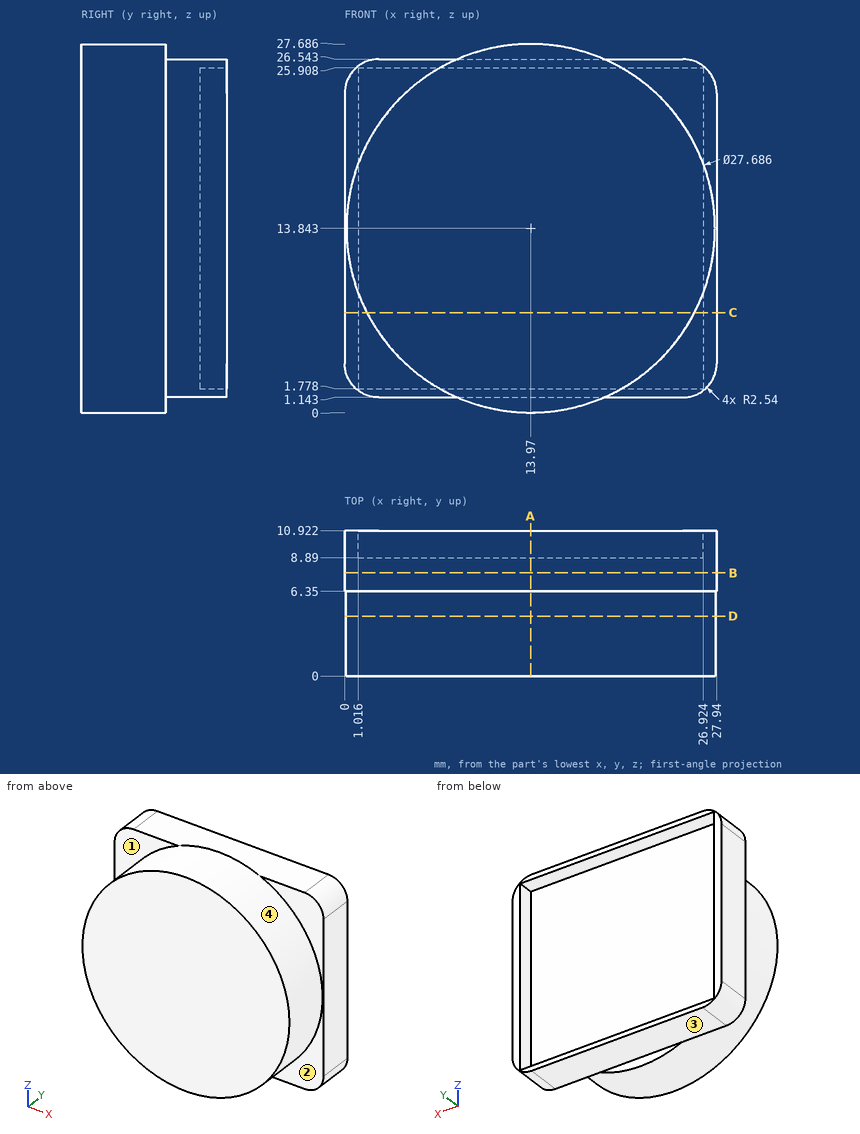
For this review, use the dimensioned drawing (mm, ordinates from the lowest corner) and the shaded views. A direction names the side the tool comes from. Round coordinates to 2 decimals unless told otherwise and drop trailing zeros. Order: outer loops, then holes, each group sorted by start corner. A loop starts at its lowest first (then second) coordinate and runs counter-clockwise, first axis right, second up. Notation, with made-up numbers: M 86.25,-29 L 101.25,-29 A22 cw 101.25,-21 Z; hole C 77,26 d11. An arc over 180 degrees is marked long. Write each question's results on one line, items separated by ' | '. Start each with the question number.
1. Add section B-B (y = 7.75). State the section outline as (x, z) points.
2. To check wall thickness, follow L1, parallel to Z at x = 24.25, y = 6.5; L2, parallel to X at y = 10, z = 19.5; L3, parallel to Y at x = 23.75, z = 3. State the ranges of each line that lie inside material, in increasing order. Write a range as [from, to].
3. Add section C-C (z = 7.5). State the section outline as (x, y) points.
4. Add section D-D (y = 4.5). State the section outline as (x, z) points, then the cut area to 3 significant figures.
5. Tool access review of the marked faces 1, 2, 3 and 4: name each direction out of +Z, -Z, +X, -X, +Y, -Y from which nothing blocks a thin tool from reaching the whole face with its end or side.
6. Add section A-A (x = 13.97). State the section outline as (y, z) points.
7. Clearance check with flat-ended pins moving along their axes: pin 1 Ø1.4 at (x, y) = (8.5, 8.5) entering from +Z; pin 2 Ø4 at (x, z) = (3.5, 23) entering from +Y; pin 3 Ø1.4 at (x, y) = (18.5, 8) entering from -Z. State where each tip first meets the part, or that it passes through.
Output values:
1) outline: M 0,3.68 A2.54 ccw 2.54,1.14 L 25.4,1.14 A2.54 ccw 27.94,3.68 L 27.94,24 A2.54 ccw 25.4,26.54 L 2.54,26.54 A2.54 ccw 0,24 Z
2) L1: [1.14, 26.54] | L2: [0, 1.02], [26.92, 27.94] | L3: [6.35, 8.89]
3) outline: M 0,6.35 L 1.67,6.35 L 1.67,0 L 26.27,0 L 26.27,6.35 L 27.94,6.35 L 27.94,10.92 L 26.92,10.92 L 26.92,8.89 L 1.02,8.89 L 1.02,10.92 L 0,10.92 Z
4) outline: C 13.97,13.84 d27.69 | area: 602 mm^2
5) face 1: -X, -Y | face 2: +X, -Y | face 3: -Z, +X, -X, +Y | face 4: -Y
6) outline: M 0,0 L 6.35,0 L 6.35,1.14 L 10.92,1.14 L 10.92,1.78 L 8.89,1.78 L 8.89,25.91 L 10.92,25.91 L 10.92,26.54 L 6.35,26.54 L 6.35,27.69 L 0,27.69 Z
7) pin 1: z = 26.54 | pin 2: y = 8.89 | pin 3: z = 1.14
